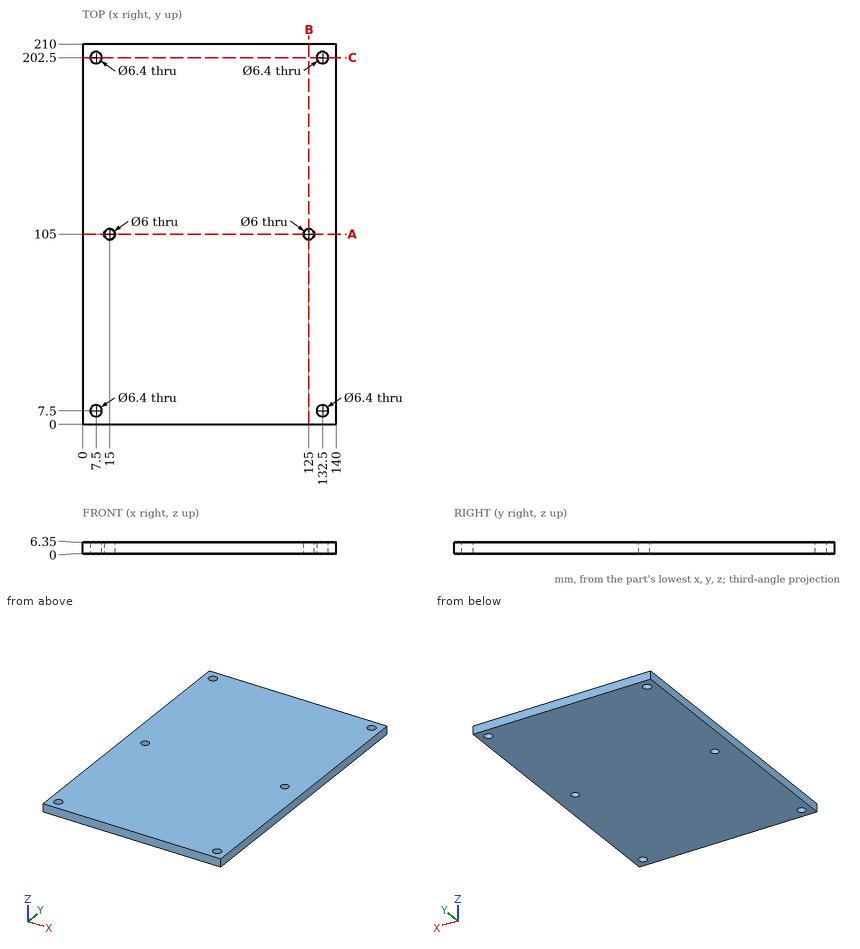
Source: three-view drawing plus pictorial views. Frame: mm from the lowest corner of the part. Coordinates: 2 decimals unless noted, no trailing zeros. Order: outer loops, then holes, each group sorted by start corner. A loop starts at its lowest first (then second) coordinate and runs counter-clockwise, first axis right, second up. Notation, with made-up numbers: M -18.75,18 L -0.75,18 A24 ccw -0.75,37 Z; hole C 69,72.25 d7. An arc over 180 degrees is marked long. Write each question's results on one line, items separated by ' | '. Start each with the question number.
1. Material intervals for L1, parallel to X at y = 105, z = 2.5; L2, parallel to Y at x = 132.5, z = 2; L3, parallel to X at y = 7.5, z = 3, sorted ascending.
2. Section B-B, the plane x = 125. Return the cut outline in (y, z), then the cut area to 3 significant figures.
3. Section C-C, the plane y = 202.5. Return the cut outline in (x, z).
4. Section A-A, the plane y = 105. Return the cut outline in (x, z), then the cut area to 3 significant figures.
Solution:
1) L1: 0 to 12, 18 to 122, 128 to 140 | L2: 0 to 4.3, 10.7 to 199.3, 205.7 to 210 | L3: 0 to 4.3, 10.7 to 129.3, 135.7 to 140
2) outline: M 0,0 L 102,0 L 102,6.35 L 0,6.35 Z; M 108,0 L 210,0 L 210,6.35 L 108,6.35 Z | area: 1,300 mm²
3) outline: M 0,0 L 4.3,0 L 4.3,6.35 L 0,6.35 Z; M 10.7,0 L 129.3,0 L 129.3,6.35 L 10.7,6.35 Z; M 135.7,0 L 140,0 L 140,6.35 L 135.7,6.35 Z
4) outline: M 0,0 L 12,0 L 12,6.35 L 0,6.35 Z; M 18,0 L 122,0 L 122,6.35 L 18,6.35 Z; M 128,0 L 140,0 L 140,6.35 L 128,6.35 Z | area: 813 mm²
